The drawing under review shows one solid part. Ordinate dimensions are in mm from its lowest x, y, z. A direction names the side the tool comes from. Give positions to 0.01 mm unless a question says otherwise; leave off trailing zeros. Write each loop counter-clockwise with the first axis right and the second up, starting at its lowest first coordinate (ties: lowest second). Pieces come first, ordered by that corner, then holes. Notation, with made-up numbers: (-15, 75.25) -> (40, 75.25) arc R32 ccw to (40, 111.25) -> close; hole circle Ø8 at (-2.5, 34). An arc over 180 degrees is marked (long way). Answer as a JSON object with one key per item and string values.
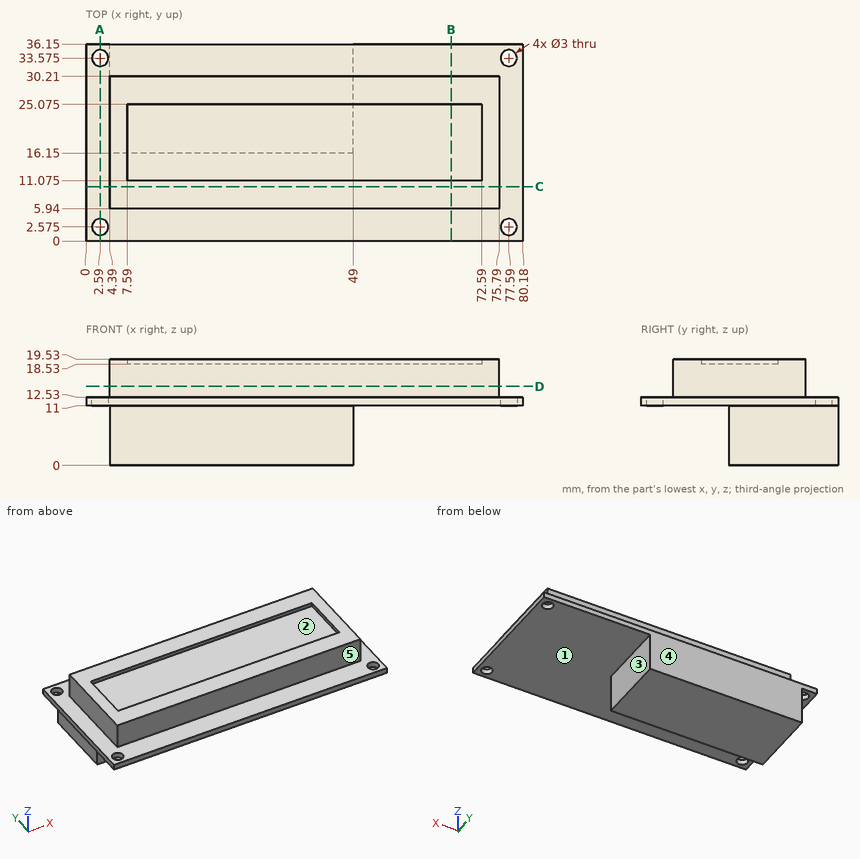
(1) We need section C-C, the plane y = 10. State the section outline as (x, z) points.
Here are the results:
{"outline": "(0, 11) -> (80.18, 11) -> (80.18, 12.53) -> (75.79, 12.53) -> (75.79, 19.53) -> (4.39, 19.53) -> (4.39, 12.53) -> (0, 12.53) -> close"}
(2) We need section B-B, the plane x = 67. State the section outline as (y, z) points (3 decimals), then the cut area to 3 significant figures.
Here are the results:
{"outline": "(0, 11) -> (36.15, 11) -> (36.15, 12.53) -> (30.21, 12.53) -> (30.21, 19.53) -> (25.075, 19.53) -> (25.075, 18.53) -> (11.075, 18.53) -> (11.075, 19.53) -> (5.94, 19.53) -> (5.94, 12.53) -> (0, 12.53) -> close", "area": "211 mm²"}
(3) We need section A-A, the plane x = 2.59. State the section outline as (y, z) points (3 decimals), then the cut area to 3 significant figures.
Here are the results:
{"outline": "(0, 11) -> (1.075, 11) -> (1.075, 12.53) -> (0, 12.53) -> close; (4.075, 11) -> (32.075, 11) -> (32.075, 12.53) -> (4.075, 12.53) -> close; (35.075, 11) -> (36.15, 11) -> (36.15, 12.53) -> (35.075, 12.53) -> close", "area": "46.1 mm²"}
(4) Clearance check with flat-ended pins moving along their axes: pin 1 (4 mm diameter, centred on x = 68, z = 15.5, fed in from -Y); pin 2 (6 mm diameter, centred on x = 56.5, z = 13.5, fed in from -Y); pin 3 (3.5 mm diameter, centred on y = 20.5, z = 17.5, fed in from -X); pin 4 (3.5 mm diameter, centred on x = 29, z = 5.5, fed in from -Y). State where each tip first meets the part, or that it passes through.
Here are the results:
{"pin 1": "stops at y = 5.94", "pin 2": "stops at y = 0", "pin 3": "stops at x = 4.39", "pin 4": "stops at y = 16.15"}
(5) For line 1 along Y through (x, z) = (2.59, 11.85) (3 decimals); line 2 along X through (y, z) = (16.5, 13); line 3 along Z through (x, y) = (26.5, 23.5), list the stretches that pass through material, from the lowest coordinate up.
Here are the results:
{"line 1": "y = 0 to 1.075, 4.075 to 32.075, 35.075 to 36.15", "line 2": "x = 4.39 to 75.79", "line 3": "z = 0 to 18.53"}
(6) For the marked faces 4 and 5, list the 3-axis set-ups (+Z, -Z, +X, -X, +Y, -Y) from which the entire face can be reached by the end or side of a thin tool; tool diameter is ignored.
Here are the results:
{"face 4": "+Z, -Z, +X, -X, +Y", "face 5": "+Z, +X, -X, -Y"}
(7) The part is to be moulded in two halves that separate along X. For the marked faces 1, 2 and 3, say which applies: +X half, -X half, draft (parallel to the pull), parting line (faces both ways), or undercut.
Here are the results:
{"face 1": "draft", "face 2": "undercut", "face 3": "+X half"}
(8) We need section D-D, the plane z = 14.5. State the section outline as (x, y) points, then the cut area to 3 significant figures.
Here are the results:
{"outline": "(4.39, 5.94) -> (75.79, 5.94) -> (75.79, 30.21) -> (4.39, 30.21) -> close", "area": "1,730 mm²"}
